Read the model definition and answer for the solid it produces. Units are mm, in the model's axes. Face numbers are marked on the shaded views. Round coordinates to 2 decimals unless told otherwise and drop trailing zeros. Write each loop counter-clockwise with the first axis right and the second up, starting at its lowest first coordinate (ties: lowest second). Pieces come first, ordered by that corner, then holes.
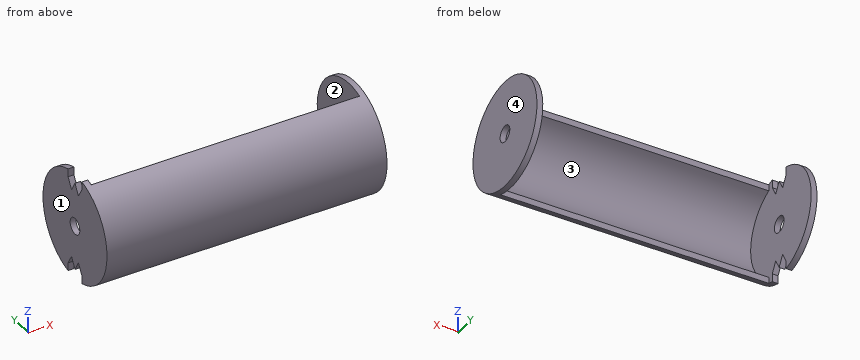
from build123d import *

# Parameters (mm, degrees)
SKETCH1_R               = 58.7375
SKETCH1_R_2             = 8.89
BOSS_EXTRUDE1_DEPTH     = 152.4
CUT_EXTRUDE1_DEPTH      = 174.568279972
CUT_EXTRUDE1_DEPTH_BACK = 174.568279972
SKETCH2_W               = 292.1
SKETCH2_H               = 77.7875
SHELL1_START            = -146.05
SHELL1_DEPTH            = 292.1
CUT_EXTRUDE2_DEPTH      = 12.7


# Read off the part's stored shape, not the designer's step: Shell1
with BuildPart() as part:
    # Sketch1 → Boss-Extrude1 (new, symmetric)
    with BuildSketch(Plane(origin=(0, 0, 0), x_dir=(0, 0, -1), z_dir=(1, 0, 0))):
        with Locations(Location((0, 0, 0), (0, 0, 180))):
            Circle(SKETCH1_R)
        with Locations(Location((0, 0, 0), (0, 0, 180))):
            Circle(SKETCH1_R_2, mode=Mode.SUBTRACT)
    extrude(amount=BOSS_EXTRUDE1_DEPTH, both=True)

    # Sketch2 → Cut-Extrude1 (cut, two sides: drawn at the far end of the back side and taken through both)
    with BuildSketch(Plane.XY.offset(-CUT_EXTRUDE1_DEPTH_BACK)):
        with Locations((0, 19.84375)):
            Rectangle(SKETCH2_W, SKETCH2_H)
    extrude(amount=CUT_EXTRUDE1_DEPTH + CUT_EXTRUDE1_DEPTH_BACK, mode=Mode.SUBTRACT)

    # Shell1 outline → Shell1 (cut)
    with BuildSketch(Plane.YZ.offset(SHELL1_START)):
        with BuildLine():
            ThreePointArc((-19.05, 48.801103023), (-52.3875, 0), (-19.05, -48.801103023))
            Line((-19.05, -48.801103023), (-19.05, 48.801103023))
        make_face()
    extrude(amount=SHELL1_DEPTH, mode=Mode.SUBTRACT)

    # Sketch3 → Cut-Extrude2 (cut)
    with BuildSketch(Plane.ZY.offset(152.4)):
        Polygon((-48.5775, 12.7), (-37.578977372, 6.35), (-48.5775, 0), (-37.578977372, -6.35), (-48.5775, -12.7), (-58.7375, -12.7), (-58.7375, 12.7), align=None)
        Polygon((48.5775, 12.7), (58.7375, 12.7), (58.7375, -12.7), (48.5775, -12.7), (37.578977372, -6.35), (48.5775, 0), (37.578977372, 6.35), align=None)
    extrude(amount=-CUT_EXTRUDE2_DEPTH, mode=Mode.SUBTRACT)


solid = part.part
Q1. Straight lines are drawn through the part: probe 1 along X at (y, z) = (-46, 6); probe 2 along Y at (x, z) = (149, 0); probe 3 along Y at (x, z) = (13, 1). For each, find the intervals that lie inside material, in ascending order.
Verdict:
probe 1: x = -152.4 to -146.05, 146.05 to 152.4
probe 2: y = -58.74 to -8.89, 8.89 to 58.74
probe 3: y = -58.73 to -52.38
Q2. Section A-A (z = 0) is taken. Determine the outline of the cut face in (x, y).
Verdict:
outline: (-152.4, -58.74) - (152.4, -58.74) - (152.4, -8.89) - (146.05, -8.89) - (146.05, -52.39) - (-146.05, -52.39) - (-146.05, -8.89) - (-152.4, -8.89) - close; (-152.4, 8.89) - (-146.05, 8.89) - (-146.05, 58.74) - (-152.4, 58.74) - close; (146.05, 8.89) - (152.4, 8.89) - (152.4, 58.74) - (146.05, 58.74) - close
Q3. Section C-C (z = -18) is taken. Determine the outline of the cut face in (x, y), then the cut area to 3 significant figures.
Verdict:
outline: (-152.4, -55.91) - (152.4, -55.91) - (152.4, 55.91) - (146.05, 55.91) - (146.05, -49.2) - (-146.05, -49.2) - (-146.05, 55.91) - (-152.4, 55.91) - close
area: 3,380 mm2
Q4. Section B-B (y = -33) is taken. Determine the outline of the cut face in (x, z), then the cut area to 3 significant figures.
Verdict:
outline: (-152.4, -48.59) - (152.4, -48.59) - (152.4, 48.59) - (-152.4, 48.59) - close; hole (-146.05, -40.69) - (146.05, -40.69) - (146.05, 40.69) - (-146.05, 40.69) - close
area: 5,850 mm2
Q5. Determine the mould class of the marked faces 1, 2, 3 and 4 for opening direction X: pulls with the +X half, pulls with the -X half, needs draft (parallel to the pull), parting line crosses it, or undercut.
Verdict:
face 1: pulls with the -X half
face 2: undercut
face 3: undercut
face 4: pulls with the +X half
Q6. Flat-ended cylindrical pins translate along their axes: pin 1 Ø1.9 at (x, z) = (-149.5, -54.5) entering from +Y; pin 2 Ø2 at (x, z) = (-88.5, -18) entering from -Y; pin 3 Ø1.9 at (x, z) = (-149, 53) entering from -Y. Find the tip coordinate at first contact, or state that the pin passes through.
Verdict:
pin 1: stops at y = 24.13
pin 2: stops at y = -56.22
pin 3: stops at y = -27.22
